CAD build for the part. Positions are in the model's coordinates, mm. A direction names the side the tool comes from. Coordinates: 2 decimals unless noted, no trailing zeros. Loops run counter-clockwise (first coordinate to the right, second up) from the corner with the lowest first, then second, coordinate; pieces in that order, holes last. Notation, with made-up numbers: (58, -35) -> (109, -35) arc R30 ccw to (109, -1) -> close; hole circle Ø5 at (-19.75, -5.75). An arc over 180 degrees is marked (long way). Write each question's results on one line, items separated by ' | '.
Autodesk Inventor part; units mm, degrees
ref_plane "YZ Plane" through (0, 0, 0) normal (1, 0, 0) x (0, 1, 0)
ref_plane "XZ Plane" through (0, 0, 0) normal (0, 1, 0) x (-1, 0, 0)
ref_plane "XY Plane" through (0, 0, 0) normal (0, 0, 1) x (1, 0, 0)
sketch "Sketch1" plane through (0, 0, 0) normal (0, 1, 0) x (-1, 0, 0)
  circle A0 centre (0, 0) radius 8 construction
  circle A1 centre (0, 0) radius 2.35
  line L0 (30, 15) -> (-30, 15)
  line L1 (-30, 15) -> (-30, -15)
  line L2 (-30, -15) -> (30, -15)
  line L3 (30, -15) -> (30, 15)
  line L4 (0, -21) -> (0, 21)
  point P0 (0, 15)
  dimension "d0" = 16
  dimension "d3" = 4.7
  dimension "d4" = 60
  dimension "d5" = 30
  dimension "d6" = 15
extrude "Extrusion1" add sketch "Sketch1" along normal blind 2.5 contours A1 L4 L0 L3 L2 | A1 L4 L2 L1 L0
sketch "Sketch2" plane through (0, 2.5, 0) normal (0, 1, 0) x (1, 0, 0)
  circle A0 centre (0, 0) radius 3.5
  line L0 (-30, 15) -> (-30, -15)
  line L1 (-30, -15) -> (30, -15)
  line L2 (30, -15) -> (30, 15)
  line L3 (30, 15) -> (-30, 15)
  circle A1 centre (0, 0) radius 2.35
  dimension "d9" = 7
extrude "Extrusion2" add sketch "Sketch2" along normal blind 1 contours L3 L2 L1 L0
sketch "Sketch4" plane through (0, 0, 0) normal (0, -1, 0) x (1, 0, 0)
  line L0 (-42, 0) -> (42, 0)
  point P0 (0, 0)
  point P1 (-5.5, 0)
  point P2 (5.5, 0)
  dimension "d18" = 360
  dimension "d20" = 5.5
hole "Hole1" at (-5.5, 0, 0) at (5.5, 0, 0) direction (0, 1, 0) diameter 2.4 end through all counterbore diameter 4.4 counterbore depth 2.3
sketch "Sketch5" plane through (0, 2.5, 0) normal (0, 1, 0) x (1, 0, 0)
  circle A0 centre (0, 0) radius 8
  dimension "d30" = 16
extrude "Extrusion3" cut sketch "Sketch5" along normal blind 1
sketch "Sketch7" plane through (0, 0, 0) normal (0, -1, 0) x (1, 0, 0)
  circle A0 centre (-25, 10) radius 4
  line L0 (-30, 15) -> (30, 15)
  line L1 (-30, -15) -> (-30, 15)
  circle A1 centre (25, 10) radius 4
  circle A2 centre (-25, -10) radius 4
  circle A3 centre (25, -10) radius 4
  point P0 (0, 0)
  dimension "d34" = 8
  dimension "d35" = 5
  dimension "d36" = 5
  dimension "d39" = 50
  dimension "d42" = 20
extrude "Extrusion4" cut sketch "Sketch7" against normal blind 1
chamfer "Chamfer1" distance 0.25 angle 45 1 edges at (2.35, 2.5, 0)
sketch "Sketch9" plane through (0, 3.5, 0) normal (0, 1, 0) x (1, 0, 0)
  circle A0 centre (-25, -10) radius 4 construction
  point P0 (0, 0)
hole "Hole2" at (-25, 3.5, 10) direction (0, -1, 0) diameter 3.4 end through all
pattern_linear "Rectangular Pattern1" count 2 spacing 20 along (0, 0, -1) count 2 spacing 50 along (1, 0, 0) of "Hole2"
sketch "Sketch10" plane through (5.5, 2.3, 0) normal (0, -1, 0) x (1, 0, 0)
  circle A0 centre (0, 0) radius 2.2
  circle A1 centre (0, 0) radius 1.2
  circle A2 centre (-11, 0) radius 2.2
  circle A3 centre (-11, 0) radius 1.2
  point P0 (-5.5, 0)
extrude "Extrusion6" add sketch "Sketch10" along normal blind 1
properties part number "motor mount plate"
1) Which spindle directions (+Z, -Z, +X, -X, +Y, -Y) get a long thin tool onto all of the face, cutting with end or side? Do faces 4 (the cylindrical face through (-1.73, 2.99, -7.81)), 5 (the flat face through (-23, 1, -10)), 6 (the cylindrical face through (-4.386, 1.908, -0.447)). Say none if no direction does.
Outcome:
face 4: +Y | face 5: -Y | face 6: +Y, -Y
2) Two-plate mould, pull along Z, no slides. Class faces 1 (the flat face through (27, 1, 10)), 2 (the flat face through (0, 2, 15)), 3 (the flat face through (-30, 2, 0)): pulls with the +Z half, pulls with the -Z half, needs draft (parallel to the pull), parting line crosses it, or undercut.
Outcome:
face 1: undercut | face 2: pulls with the +Z half | face 3: needs draft
3) Drill centre lines: L1, parallel to Z at x = -25, y = 2.45; L2, parallel to X at y = 2.5, z = 10; L3, parallel to X at y = 1.85, z = -10.5. Where is each one in solid material? Low to high. Write a range as from..to.
Outcome:
L1: z = -15..-11.7, -8.3..8.3, 11.7..15 | L2: x = -30..-26.7, -23.3..23.3, 26.7..30 | L3: x = -30..-26.62, -23.38..23.38, 26.62..30
4) Slice it at D-D (x = 5.5). Write the cut outline in (y, z), then the cut area to 3 significant figures.
Outcome:
outline: (0, -15) -> (3.5, -15) -> (3.5, -5.81) -> (2.5, -5.81) -> (2.5, -1.2) -> (1.3, -1.2) -> (1.3, -2.2) -> (0, -2.2) -> close; (0, 2.2) -> (1.3, 2.2) -> (1.3, 1.2) -> (2.5, 1.2) -> (2.5, 5.81) -> (3.5, 5.81) -> (3.5, 15) -> (0, 15) -> close | area: 84.8 mm^2
5) Slice it at A-A (x = -25). Write the cut outline in (y, z).
Outcome:
outline: (0, -15) -> (3.5, -15) -> (3.5, -11.7) -> (1, -11.7) -> (1, -14) -> (0, -14) -> close; (0, -6) -> (1, -6) -> (1, -8.3) -> (3.5, -8.3) -> (3.5, 8.3) -> (1, 8.3) -> (1, 6) -> (0, 6) -> close; (0, 14) -> (1, 14) -> (1, 11.7) -> (3.5, 11.7) -> (3.5, 15) -> (0, 15) -> close
6) Slice it at B-B (z = 0). Count the separate pieces of the cut face and the enclosed holes in it, then the cut area to 3 significant figures.
Outcome:
separate pieces: 4 | enclosed holes: 0 | area: 165 mm^2
7) Slice it at C-C (z = -10). Write the cut outline in (x, y).
Outcome:
outline: (-30, 0) -> (-29, 0) -> (-29, 1) -> (-26.7, 1) -> (-26.7, 3.5) -> (-30, 3.5) -> close; (-23.3, 1) -> (-21, 1) -> (-21, 0) -> (21, 0) -> (21, 1) -> (23.3, 1) -> (23.3, 3.5) -> (-23.3, 3.5) -> close; (26.7, 1) -> (29, 1) -> (29, 0) -> (30, 0) -> (30, 3.5) -> (26.7, 3.5) -> close
8) Pin check, flat tips, straight feed: pin 1 (2 mm diameter, centred on x = 25, z = 10, fed in from +Y); pin 2 (6.5 mm diameter, centred on x = -24.5, z = 9.5, fed in from -Y); pin 3 (4 mm diameter, centred on x = -5.5, z = 0, fed in from -Y); pin 4 (8 mm diameter, centred on x = 0.5, z = -2.5, fed in from +Y). Stop position of each tip, or through.
Outcome:
pin 1: passes through | pin 2: stops at y = 1 | pin 3: stops at y = 1.3 | pin 4: stops at y = 2.5
